Geometry check sheet. Reference: the model listing, model coordinates, mm. Face numbers are marked on the shaded views. Coordinates: 2 decimals unless noted, no trailing zeros. Loops run counter-clockwise (first coordinate to the right, second up) from the corner with the lowest first, then second, coordinate; pieces in that order, holes last. Notation, with made-up numbers: (80, 80) - (118, 80) arc R4 cw to (118, 87) - close; hole circle Ø4 at (12.5, -26.75). An arc over 180 degrees is marked (long way). Write item = value, one per line. Start each with the question number.
from build123d import *

# Parameters (mm, degrees)
F1_DEPTH = 5
F2_R     = 0.3


with BuildPart() as f1:
    # F0 (on Top) → F1 (new body)
    with BuildSketch(Plane.XY):
        with BuildLine():
            ThreePointArc((-4.935585, 0.8), (0, 5), (4.935585, 0.8))
            Line((4.935585, 0.8), (0.987117, 25.16))
            ThreePointArc((0.987117, 25.16), (0, 26), (-0.987117, 25.16))
            Line((-0.987117, 25.16), (-4.935585, 0.8))
        make_face()
        with BuildLine():
            ThreePointArc((-4.935585, 0.8), (-0.401295, -4.98387), (5, 0))
            ThreePointArc((5, 0), (4.98387, 0.401295), (4.935585, 0.8))
            ThreePointArc((4.935585, 0.8), (0, 5), (-4.935585, 0.8))
        make_face()
        with BuildLine():
            ThreePointArc((1.5, 2), (2.236068, 1.118034), (2.5, 0))
            ThreePointArc((2.5, 0), (-1.118034, -2.236068), (-1.5, 2))
            ThreePointArc((-1.5, 2), (0, 2.5), (1.5, 2))
        make_face(mode=Mode.SUBTRACT)
        with BuildLine():
            Line((-1.5, 2), (1.5, 2))
            ThreePointArc((1.5, 2), (0, 2.5), (-1.5, 2))
        make_face()
    extrude(amount=F1_DEPTH)

    # F2
    f2_edges = [f1.edges().sort_by_distance(p)[0] for p in [
        (-0.401295, -4.98387, 5),
        (4.98387, 0.401295, 5),
        (2.961351, 12.98, 5),
        (0, 26, 5),
        (-2.961351, 12.98, 5),
        (0, -2.5, 5),
        (0, 2, 5),
        (4.98387, 0.401295, 0),
        (2.961351, 12.98, 0),
        (0, 26, 0),
        (-2.961351, 12.98, 0),
        (-0.401295, -4.98387, 0),
        (0, -2.5, 0),
        (0, 2, 0),
    ]]
    fillet(f2_edges, radius=F2_R)


solid = f1.part
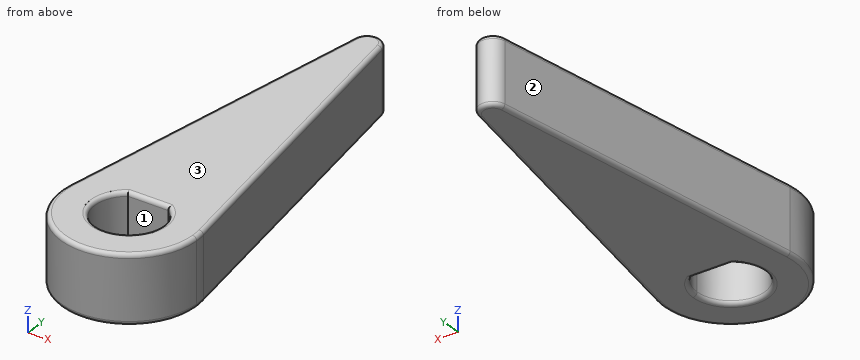
(1) Draft check along Y on the marked faces 1, 2 and 3. Enter one of: pulls with the +Y half, pulls with the -Y half, needs draft (parallel to the pull), parting line crosses it, or undercut.
(2) Scan lines: line 1 (Y direction, x = 0, z = 1.9); line 2 (Y direction, x = -0.5, z = 2.55); line 3 (Z direction, x = 4.25, y = 3.5). Record each from-to range of solid material in increasing order.
(3) Sectioned sample at A-A on z = 1.6. Enter the section's corners in (x, y).
Working result:
q1.face_1 = undercut
q1.face_2 = pulls with the +Y half
q1.face_3 = needs draft
q2.line_1 = -5 to -2.5, 2 to 26
q2.line_2 = -4.97 to -2.45, 2 to 25.87
q2.line_3 = 0.01 to 4.99
q3.outline = (-4.94, 0.8) arc R5 ccw (long way) to (5, 0) arc R5 ccw to (4.94, 0.8) - (0.99, 25.16) arc R1 ccw to (-0.99, 25.16) - close; hole (-1.5, 2) arc R2.5 ccw (long way) to (1.5, 2) - close
